Geometry: final body of the model. Coordinates: model frame, mm. A direction names the side the tool comes from. Round coordinates to 2 decimals unless told otherwise and drop trailing zeros. Loops run counter-clockwise (first coordinate to the right, second up) from the corner with the lowest first, then second, coordinate; pieces in that order, holes last. Notation, with made-up numbers: M 35.25,25 L 84.25,25 A21 ccw 84.25,34 Z; hole C -10.5,41.5 d1. An arc over 180 degrees is marked long. Answer as a JSON object with one key per item and string values.
```python
from build123d import *

# Parameters (mm, degrees)
SKETCH1_W                        = 152.4
SKETCH1_H                        = 88.9
BOSS_EXTRUDE1_DEPTH              = 6.35
F_17_64_0_26563_DIAMETER_HOLE1_D = 6.747002
LPATTERN1_COUNT                  = 4
LPATTERN1_PITCH                  = 38.1
LPATTERN1_COUNT_DIR2             = 2
LPATTERN1_PITCH_DIR2             = 38.1
SKETCH4_W                        = 76.2
SKETCH4_H                        = 12.7
CUT_EXTRUDE1_DEPTH               = 177.548272436
FILLET1_R                        = 6.35


with BuildPart() as part:
    # Sketch1 → Boss-Extrude1 (new body)
    with BuildSketch(Plane.XY):
        with Locations((76.2, 44.45)):
            Rectangle(SKETCH1_W, SKETCH1_H)
    extrude(amount=BOSS_EXTRUDE1_DEPTH)

    # 17/64 (0.26563) Diameter Hole1 (through all)
    with Locations(Plane.XY.offset(6.35)):
        with Locations((19.05, 19.05)):
            f_17_64_0_26563_diameter_hole1 = Hole(F_17_64_0_26563_DIAMETER_HOLE1_D / 2)

    # LPattern1: 17_64 _0.26563_ Diameter Hole1 4 × 2
    with Locations(*[(i * LPATTERN1_PITCH, j * LPATTERN1_PITCH_DIR2, 0) for i in range(LPATTERN1_COUNT) for j in range(LPATTERN1_COUNT_DIR2) if (i, j) != (0, 0)]):
        add(f_17_64_0_26563_diameter_hole1, mode=Mode.SUBTRACT)

    # Sketch4 → Cut-Extrude1 (cut, through all)
    with BuildSketch(Plane.XY.offset(6.35)):
        with Locations((114.3, 82.55)):
            Rectangle(SKETCH4_W, SKETCH4_H)
    extrude(amount=-CUT_EXTRUDE1_DEPTH, mode=Mode.SUBTRACT)

    # Fillet1
    fillet1_edges = [part.edges().sort_by_distance(p)[0] for p in [
        (76.2, 76.2, 3.175),
    ]]
    fillet(fillet1_edges, radius=FILLET1_R)


solid = part.part
```
1) Cut plane C-C on z = 2.25. Count the separate pieces of the cut face and the enclosed holes in it, and give its area (3 significant figures).
Geometry results:
{"separate pieces": "1", "enclosed holes": "8", "area": "12,300 mm2"}
2) Cut plane B-B on x = 95.25. Return the cut outline in (y, z), and give its area (3 significant figures).
Geometry results:
{"outline": "M 0,0 L 15.68,0 L 15.68,6.35 L 0,6.35 Z; M 22.42,0 L 53.78,0 L 53.78,6.35 L 22.42,6.35 Z; M 60.52,0 L 76.2,0 L 76.2,6.35 L 60.52,6.35 Z", "area": "398 mm2"}
3) Pull-direction query (X, two-part tool) for faces 1 (the face through (130.13, 20.06, 3.13)), 2 (the face through (75, 0, 3)), 3 (the face through (76.2, 86, 3)), 4 (the face through (95.689, 60.495, 3.131)); classes: +X half, -X half, draft (parallel to the pull), parting line (faces both ways), or undercut.
Geometry results:
{"face 1": "undercut", "face 2": "draft", "face 3": "+X half", "face 4": "undercut"}
4) Set-up query: faces 5 (the face through (117, 76.2, 3)), 6 (the face through (19.489, 60.495, 3.131)). Return all of +Z, -Z, +X, -X, +Y, -Y with unobstructed straight access to the full face (end or side cutting, diameter ignored); none if empty.
Geometry results:
{"face 5": "+Z, -Z, +X, +Y", "face 6": "+Z, -Z"}
5) Cut plane D-D on x = 19.05. Return the cut outline in (y, z).
Geometry results:
{"outline": "M 0,0 L 15.68,0 L 15.68,6.35 L 0,6.35 Z; M 22.42,0 L 53.78,0 L 53.78,6.35 L 22.42,6.35 Z; M 60.52,0 L 88.9,0 L 88.9,6.35 L 60.52,6.35 Z"}
6) Line query: probe 1 along Y at (x, z) = (57, 1.75); probe 2 along X at (y, z) = (60, 4) (3 decimals); probe 3 along X at (y, z) = (21.5, 5.25). Output: solid intervals per line, ascending.
Geometry results:
{"probe 1": "0 to 15.68, 22.42 to 53.78, 60.52 to 88.9", "probe 2": "0 to 17.245, 20.855 to 55.345, 58.955 to 93.445, 97.055 to 131.545, 135.155 to 152.4", "probe 3": "0 to 16.73, 21.37 to 54.83, 59.47 to 92.93, 97.57 to 131.03, 135.67 to 152.4"}
7) Cut plane A-A on y = 19.05. Return the cut outline in (x, z).
Geometry results:
{"outline": "M 0,0 L 15.68,0 L 15.68,6.35 L 0,6.35 Z; M 22.42,0 L 53.78,0 L 53.78,6.35 L 22.42,6.35 Z; M 60.52,0 L 91.88,0 L 91.88,6.35 L 60.52,6.35 Z; M 98.62,0 L 129.98,0 L 129.98,6.35 L 98.62,6.35 Z; M 136.72,0 L 152.4,0 L 152.4,6.35 L 136.72,6.35 Z"}
8) First-contact query: pin 1 (1.5 mm diameter, centred on x = 110, z = 5, fed in from -Y); pin 2 (5.5 mm diameter, centred on x = 133.35, y = 19.05, fed in from -Z); pin 3 (1.9 mm diameter, centred on y = 86, z = 3, fed in from +X). Flat tips, straight axial feed; report the tip coordinate or a pass-through.
Geometry results:
{"pin 1": "y = 0", "pin 2": "through", "pin 3": "x = 76.2"}
